Here's how the part is built. I have some questions about the finished solid (model axes, mm). A direction names the side the tool comes from. Give positions to 0.01 mm unless a question says otherwise; leave off trailing zeros. Use one line per item in the form item = value.
from build123d import *

# Parameters (mm, degrees)
F1_DEPTH     = 4.7625
F2_W         = 19.05
F2_H         = 6.35
F3_DEPTH     = 25.4
F4_R         = 2.54
F9_T1_DEPTH  = 9.0533559085
F9_T3_DEPTH  = 84.7725
F9_T5_DEPTH  = 53.9538612207
F9_T8_ANGLE  = 93.5585733653
F9_T10_ANGLE = 93.5585733653


# Not quite as in the source:
# - a fillet or chamfer that OpenCascade refuses, or shapes differently, is made with other operations: its cross-section is extruded or revolved along the edge and cut away or added
# - two fillets or chamfers of one size are made in one step


with BuildPart() as f1:
    # F0 (on Top) → F1 (new body, symmetric)
    with BuildSketch(Plane.XY):
        with BuildLine():
            Line((101.6, 0), (0, 0))
            Line((0, 0), (0, -50.8))
            Line((0, -50.8), (50.8, -50.8))
            ThreePointArc((50.8, -50.8), (86.7210244843, -35.9210244843), (101.6, 0))
        make_face()
    extrude(amount=F1_DEPTH, both=True)

    # F2 (on Right) → F3 (cut)
    with BuildSketch(Plane.YZ):
        with Locations((-12.7, 0)):
            Rectangle(F2_W, F2_H)
    extrude(amount=F3_DEPTH, mode=Mode.SUBTRACT)

    # F4
    f4_edges = [f1.edges().sort_by_distance(p)[0] for p in [
        (12.7, -3.175, -3.175),
        (12.7, -3.175, 3.175),
        (12.7, -22.225, -3.175),
        (12.7, -22.225, 3.175),
    ]]
    fillet(f4_edges, radius=F4_R)


with BuildPart() as f6:
    # F6: sweep along a path in F6_path
    with BuildLine(Plane(origin=(50.8, -50.8, 4.7625), x_dir=(0, 1, 0), z_dir=(0, 0, 1))) as f6_path:
        Line((0, 50.8), (0, 0))
        ThreePointArc((0, 0), (14.8789755157, -35.9210244843), (50.8, -50.8))
    # F5 (on face) → F6 (sweep)
    with BuildSketch(Plane(origin=(0, 0, 0), x_dir=(0, -1, 0), z_dir=(-1, 0, 0))):
        with BuildLine():
            Line((50.8, 4.7625), (25.4, 4.7625))
            ThreePointArc((25.4, 4.7625), (37.9805074569, 2.1472133229), (50.8, 1.27))
            Line((50.8, 1.27), (50.8, 4.7625))
        make_face()
    sweep(path=f6_path.line)


with BuildPart() as f7_1:
    # F7: instance of F6
    add(f6.part.mirror(Plane.XY))


with BuildPart() as f1_1:
    add(f1.part)

    # F8: cut F6, F7_1
    add(f6.part, mode=Mode.SUBTRACT)
    add(f7_1.part, mode=Mode.SUBTRACT)

    # F9: fillet of radius 1.27 on 8 edges, made by hand

    # F9_s2 → F9_t1 (cut)
    with BuildSketch(Plane.XY.offset(-4.5266779542)):
        with BuildLine():
            ThreePointArc((100.3137152716, 0), (101.2231811617, -0.3835623006), (101.5832977145, -1.3025641026))
            ThreePointArc((101.5832977145, -1.3025641026), (101.595824257, -0.6513355908), (101.6, 0))
            Line((101.6, 0), (100.3137152716, 0))
        make_face()
    extrude(amount=F9_T1_DEPTH, mode=Mode.SUBTRACT)

    # F9_s4 → F9_t3 (cut)
    with BuildSketch(Plane.YZ.offset(-3.175)):
        with BuildLine():
            ThreePointArc((0, 3.4925), (-0.3719743879, 4.3905256121), (-1.27, 4.7625))
            Line((-1.27, 4.7625), (0, 4.7625))
            Line((0, 4.7625), (0, 3.4925))
        make_face()
        with BuildLine():
            ThreePointArc((0, -3.4925), (-0.3719743879, -4.3905256121), (-1.27, -4.7625))
            Line((-1.27, -4.7625), (0, -4.7625))
            Line((0, -4.7625), (0, -3.4925))
        make_face()
    extrude(amount=F9_T3_DEPTH, mode=Mode.SUBTRACT)

    # F9_s6 → F9_t5 (cut)
    with BuildSketch(Plane.YZ.offset(-3.1538612207)):
        with BuildLine():
            ThreePointArc((-49.5469102739, 1.2783429251), (-50.4339845264, 0.9004824038), (-50.8, 0.0084555117))
            Line((-50.8, 0.0084555117), (-50.8, 1.27))
            ThreePointArc((-50.8, 1.27), (-50.1734412505, 1.2720857544), (-49.5469102739, 1.2783429251))
        make_face()
        with BuildLine():
            ThreePointArc((-50.8, -0.0084555117), (-50.4339845264, -0.9004824038), (-49.5469102739, -1.2783429251))
            ThreePointArc((-49.5469102739, -1.2783429251), (-50.1734412505, -1.2720857544), (-50.8, -1.27))
            Line((-50.8, -1.27), (-50.8, -0.0084555117))
        make_face()
    extrude(amount=F9_T5_DEPTH, mode=Mode.SUBTRACT)

    # F9_s7 → F9_t8 (revolve, cut)
    with BuildSketch(Plane.YZ.offset(50.8)):
        with BuildLine():
            ThreePointArc((-50.8, 0.0084555117), (-50.4339845264, 0.9004824038), (-49.5469102739, 1.2783429251))
            ThreePointArc((-49.5469102739, 1.2783429251), (-50.1734412505, 1.2720857544), (-50.8, 1.27))
            Line((-50.8, 1.27), (-50.8, 0.0084555117))
        make_face()
    revolve(axis=Axis((50.8, 0, 1.27), (0, 0, 1)), revolution_arc=F9_T8_ANGLE, mode=Mode.SUBTRACT)

    # F9_s9 → F9_t10 (revolve, cut)
    with BuildSketch(Plane.YZ.offset(50.8)):
        with BuildLine():
            ThreePointArc((-50.8, -0.0084555117), (-50.4339845264, -0.9004824038), (-49.5469102739, -1.2783429251))
            ThreePointArc((-49.5469102739, -1.2783429251), (-50.1734412505, -1.2720857544), (-50.8, -1.27))
            Line((-50.8, -1.27), (-50.8, -0.0084555117))
        make_face()
    revolve(axis=Axis((50.8, 0, -1.27), (0, 0, 1)), revolution_arc=F9_T10_ANGLE, mode=Mode.SUBTRACT)


solid = f1_1.part
(1) For faces 1 (the cylindrical face through (12.88, -3.9, -2.41)), 2 (the cylindrical face through (25.76, -37.53, 2.21)), which set-ups out of +Z, -Z, +X, -X, +Y, -Y let a thin tool reach every point of the face, with its end or its side?
Geometry says:
face_1 = -X
face_2 = +Z, +X, -X, -Y
(2) For P1, Ø1.9, axis at y = -9, z = 0.5, coming from the -X side; P2, Ø10, axis at x = 70, y = -26.5, coming from the -Z side; P3, Ø0.6, axis at x = 10, z = -0.5, coming from the -Y side, each with a flat end and sliding along its axis, tell me the tip position at first contact or that it passes through.
Geometry says:
P1 = 25.4
P2 = -4.14
P3 = -50.79
(3) If I drill on probe 1 along X at (y, z) = (-9, 1); probe 2 along Y at (x, z) = (34, -0.25); probe 3 along X at (y, z) = (-15, 1), over which ranges is the centre line in solid material (lowest first)?
Geometry says:
probe_1 = 25.4 to 100.31
probe_2 = -50.78 to 0
probe_3 = 25.4 to 98.84
(4) Thinking about a two-plate mould opening in Z: for faces 3 (the flat face through (38, -13, -4.762)), 4 (the cylindrical face through (12.88, -21.5, -2.41)), 5 (the flat face through (38, -13, 4.762)), 6 (the flat face through (0, -25, 0)), which applies, pulls with the +Z half, pulls with the -Z half, needs draft (parallel to the pull), parting line crosses it, or undercut?
Geometry says:
face_3 = pulls with the -Z half
face_4 = undercut
face_5 = pulls with the +Z half
face_6 = needs draft
